Study the drawing (mm; zero at the part's minimum x, y, z) and answer. A direction names the side the tool comes from. Coordinates: 2 decimals unless noted, no trailing zeros. Loops run counter-clockwise (first coordinate to the right, second up) from the corner with the lowest first, then second, coordinate; pieces in that order, holes last. Notation, with made-up numbers: (-7.5, 39.25) -> (45.5, 39.25) arc R32 cw to (45.5, 75.25) -> close; hole circle Ø11 at (20, 26). An arc over 180 degrees is marked (long way). One line per question, with ' | ' between items.
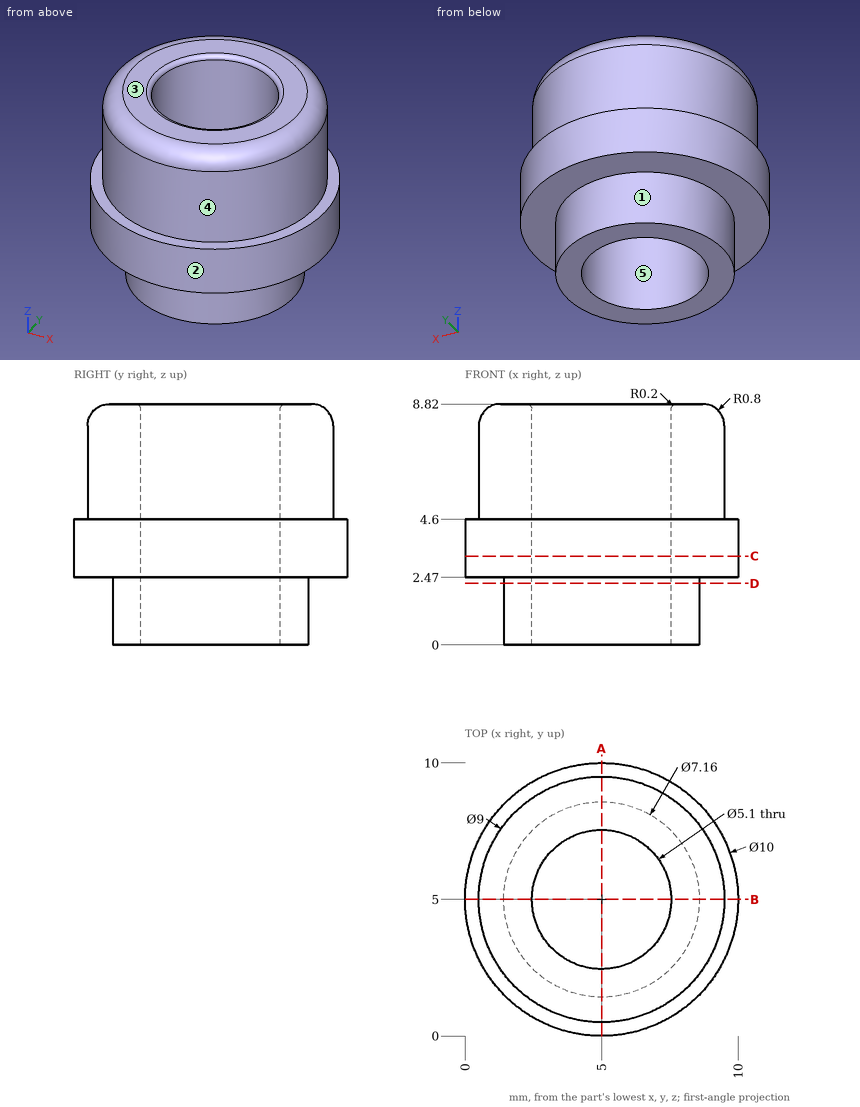
1) Flat-ended cylindrical pins translate along their axes: pin 1 (1 mm diameter, centred on y = 6, z = 3.5, fed in from -X); pin 2 (1.5 mm diameter, centred on y = 8, z = 6.5, fed in from -X); pin 3 (3 mm diameter, centred on x = 5, y = 5, fed in from -Z); pin 4 (1.5 mm diameter, centred on x = 1, z = 6.5, fed in from +Y). Find the tip coordinate at first contact, or state that the pin passes through.
Check values:
pin 1: stops at x = 0.03 | pin 2: stops at x = 1.1 | pin 3: passes through | pin 4: stops at y = 8.11
2) Find section D-D (z = 2.25). Write down the section's boundary in (x, y), plus the area to 3 significant figures.
Check values:
outline: circle Ø7.16 at (5, 5); hole circle Ø5.1 at (5, 5) | area: 19.8 mm^2
3) Find the intervals of material crossed by line 1 along Y through (x, z) = (5, 7.25); line 2 along Y through (x, z) = (5, 3.75); line 3 along Z through (x, y) = (0.5, 6.25), in increasing order.
Check values:
line 1: y = 0.5 to 2.45, 7.55 to 9.5 | line 2: y = 0 to 2.45, 7.55 to 10 | line 3: z = 2.47 to 4.6
4) The mould has two halves that part along X. Classify the marked faces 3, 4 and 5: released by +X, released by -X, zero draft, split by the parting line, or undercut.
Check values:
face 3: zero draft | face 4: split by the parting line | face 5: undercut
5) Find section C-C (z = 3.25). Write down the section's boundary in (x, y), plus the area to 3 significant figures.
Check values:
outline: circle Ø10 at (5, 5); hole circle Ø5.1 at (5, 5) | area: 58.1 mm^2
6) For the marked faces 1 and 2, determine the directions among +Z, -Z, +X, -X, +Y, -Y from which every point of the face is accessible in a straight line to the end or side of a thin tool.
Check values:
face 1: -Z | face 2: +Z, -Z
7) Find section A-A (x = 5). Write down the section's boundary in (y, z).
Check values:
outline: (0, 2.47) -> (1.42, 2.47) -> (1.42, 0) -> (2.45, 0) -> (2.45, 8.62) arc R0.2 ccw to (2.25, 8.82) -> (1.3, 8.82) arc R0.8 ccw to (0.5, 8.02) -> (0.5, 4.6) -> (0, 4.6) -> close; (7.55, 0) -> (8.58, 0) -> (8.58, 2.47) -> (10, 2.47) -> (10, 4.6) -> (9.5, 4.6) -> (9.5, 8.02) arc R0.8 ccw to (8.7, 8.82) -> (7.75, 8.82) arc R0.2 ccw to (7.55, 8.62) -> close
